For this review, take the finished solid that the model builds, in its own axes (mm). Coordinates: 2 decimals unless noted, no trailing zeros. Write each loop counter-clockwise with the first axis right and the second up, starting at its lowest first coordinate (ties: lowest second). Pieces come first, ordered by that corner, then holes. Notation, with made-up numbers: M 15,40 L 32,40 A21 ccw 32,63 Z; hole C 1,31 d1. An arc over 180 degrees is marked long. One line per question, with ' | ' between items.
Autodesk Inventor part; units mm, degrees
ref_plane "YZ Plane" through (0, 0, 0) normal (1, 0, 0) x (0, 1, 0)
ref_plane "XZ Plane" through (0, 0, 0) normal (0, 1, 0) x (-1, 0, 0)
ref_plane "XY Plane" through (0, 0, 0) normal (0, 0, 1) x (1, 0, 0)
sketch "Sketch1" plane through (0, 0, 0) normal (0, 1, 0) x (-1, 0, 0)
  line L0 (18, -21) -> (-18, -21)
  line L1 (-21, -18) -> (-21, 18)
  line L2 (-18, 21) -> (18, 21)
  line L3 (21, 18) -> (21, -18)
  line L4 (21, -21) -> (-21, 21) construction
  line L5 (-21, -21) -> (21, 21) construction
  line L6 (21, 18) -> (18, 21)
  line L7 (-21, -18) -> (-18, -21)
  line L8 (-18, 21) -> (-21, 18)
  line L9 (21, -18) -> (18, -21)
  line L10 (19.5, 19.5) -> (15.0999, 15.0999) construction
  circle A0 centre (15.5563, 15.5563) radius 1.75
  circle A1 centre (-15.5563, 15.5563) radius 1.75
  circle A2 centre (-15.5563, -15.5563) radius 1.75
  circle A3 centre (15.5563, -15.5563) radius 1.75
  circle A4 centre (0, 0) radius 11.5
  line L11 (-15.5563, 15.5563) -> (15.5563, -15.5563) construction
  dimension "d0" = 42
  dimension "d1" = 42
  dimension "d2" = 3
  dimension "d3" = 3
  dimension "d4" = 3
  dimension "d5" = 3
  dimension "d6" = 3
  dimension "d7" = 3
  dimension "d8" = 3
  dimension "d9" = 3
  dimension "d11" = 3.5
  dimension "d14" = 360
  dimension "d16" = 23
  dimension "d20" = 22
extrude "Extrusion1" add sketch "Sketch1" along normal blind 2
equation "\"d3\" = d2"
equation "\"d5\" = d4"
equation "\"d7\" = d6"
equation "\"d9\" = d8"
properties part number "washer"
1) We need section C-C on x = 14.5. State the section outline as (y, z) points.
Responses:
outline: M 0,-21 L 2,-21 L 2,-16.95 L 0,-16.95 Z; M 0,-14.16 L 2,-14.16 L 2,14.16 L 0,14.16 Z; M 0,16.95 L 2,16.95 L 2,21 L 0,21 Z
2) Insertion check: pin 1 Ø2 at (x, z) = (-15.56, -15.56) entering from -Y. The pin has a flat end and moves straight along its axis. Give the tip position at first contact, or say it passes through.
Responses:
pin 1: through
3) We need section A-A on z = 0. State the section outline as (x, y) points.
Responses:
outline: M -21,0 L -11.5,0 L -11.5,2 L -21,2 Z; M 11.5,0 L 21,0 L 21,2 L 11.5,2 Z
4) The part is to be moulded in two halves that separate along Z. For faces 1 (the flat face through (0, 1, 21)), 2 (the cylindrical face through (13.887, 0.986, -16.082)), 3 (the flat face through (10, 2, 10)), 4 (the cylindrical face through (-14.27, 0.99, -16.74)), say which applies: +Z half, -Z half, draft (parallel to the pull), parting line (faces both ways), or undercut.
Responses:
face 1: +Z half | face 2: undercut | face 3: draft | face 4: undercut
5) We need section D-D on y = 0.3. State the section outline as (x, z) points, then the cut area to 3 significant figures.
Responses:
outline: M -21,-18 L -18,-21 L 18,-21 L 21,-18 L 21,18 L 18,21 L -18,21 L -21,18 Z; hole C -15.56,-15.56 d3.5; hole C -15.56,15.56 d3.5; hole C 0,0 d23; hole C 15.56,-15.56 d3.5; hole C 15.56,15.56 d3.5 | area: 1,290 mm^2
6) To check wall thickness, follow line 1 along X through (y, z) = (1.6, -0.5); line 2 along X through (y, z) = (1.95, -16.5); line 3 along X through (y, z) = (0.9, 15). State the ranges of each line that lie inside material, in increasing order. Write a range as [from, to].
Responses:
line 1: [-21, -11.49], [11.49, 21] | line 2: [-21, -17.03], [-14.08, 14.08], [17.03, 21] | line 3: [-21, -17.22], [-13.9, 13.9], [17.22, 21]
7) We need section B-B on x = 0. State the section outline as (y, z) points, then the cut area to 3 significant figures.
Responses:
outline: M 0,-21 L 2,-21 L 2,-11.5 L 0,-11.5 Z; M 0,11.5 L 2,11.5 L 2,21 L 0,21 Z | area: 38.0 mm^2
